Check sheet for the drawn part. Datum: minimum x, y, z corner. Units: mm. A direction names the side the tool comes from. Give positions to 0.01 mm unless a question says otherwise; leave off trailing zeros. Order: outer loops, then holes, each group sorted by start corner. A loop starts at its lowest first (then second) coordinate and runs counter-clockwise, first axis right, second up. Notation, with made-up numbers: M 35.25,38 L 81.25,38 A16 ccw 81.25,65 Z; hole C 50,-11.5 d1. An arc over 180 degrees is marked long. Answer as CSV lines item,"result". Start each with the question number.
Q1. Thickness scan on line 1 (Y direction, x = 70, z = 19); line 2 (X direction, y = 58, z = 49) (3 decimals); line 3 (Z direction, x = 15.5, y = 12.5). Record the ranges inside material, lowest first.
Q2. Section check C-C, the plane z = 19.05. Record the boundary of the cut face in (x, y) (1 decimal).
Q3. Section check B-B, the plane z = 34.5. Record the boundary of the cut face in (x, y) (3 decimals), then the cut area to 3 significant figures.
Q4. Go/stop test with flat-tipped pins: pin 1 (8 mm diameter, centred on y = 34.5, z = 32.5, fed in from -X); pin 2 (4 mm diameter, centred on x = 13, y = 20.5, fed in from -Z); pin 3 (22 mm diameter, centred on x = 29.5, y = 21, fed in from -Z) (3 decimals). Record where each tip stops, or that it passes through.
Q5. Mould release check, pull along Z, two halves, no side actions. Record for the marked faces 1, 2 and 3: +Z half, -Z half, draft (parallel to the pull), parting line (faces both ways), or undercut.
Q6. Section check A-A, the plane y = 31.75. Count the separate pieces of the cut face and the enclosed holes in it, then the cut area to 3 significant figures.
Q7. Set-up check for the marked faces 4 and 5: record each of +Z, -Z, +X, -X, +Y, -Y from which the full face is reachable in a straight line by a thin tool's end or side.
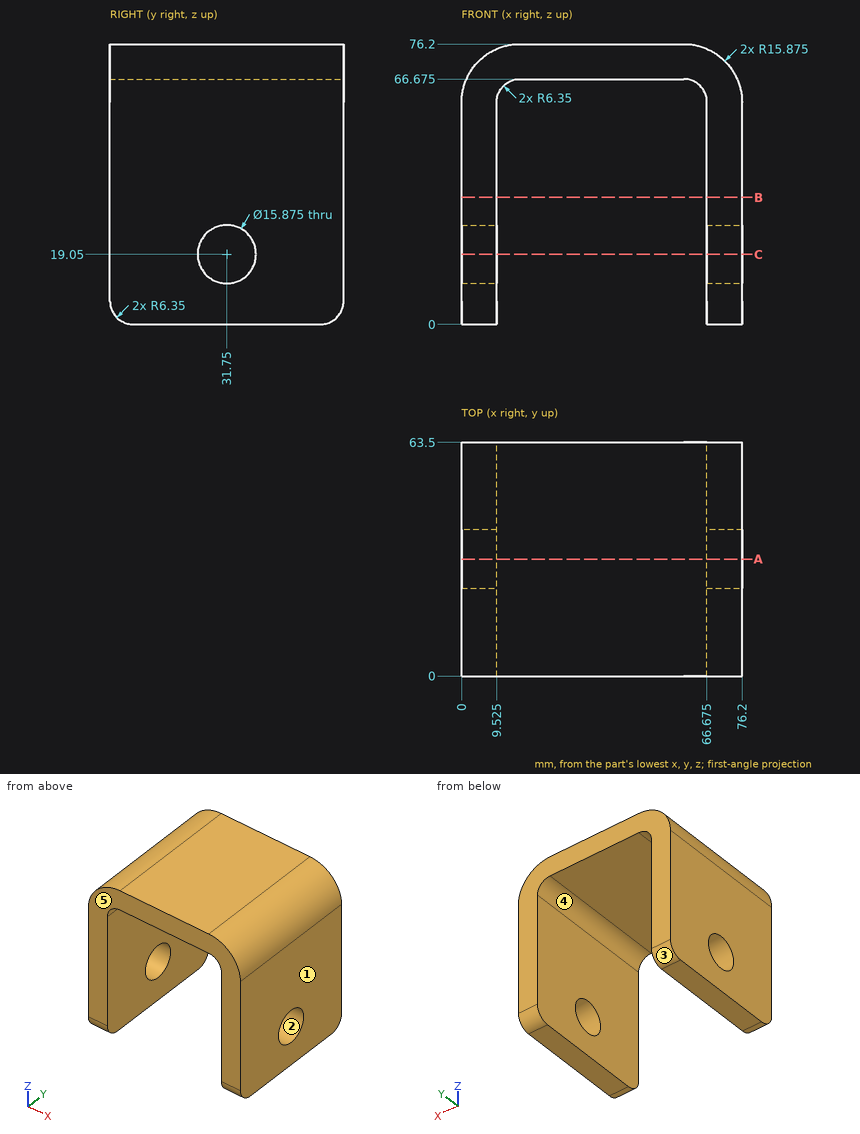
Answer block:
1,line 1,"y = 0 to 23.81, 39.69 to 63.5"
1,line 2,"x = 0 to 9.525, 66.675 to 76.2"
1,line 3,"z = 66.66 to 76.2"
2,outline,"M 0,0 L 9.5,0 L 9.5,23.8 L 0,23.8 Z; M 0,39.7 L 9.5,39.7 L 9.5,63.5 L 0,63.5 Z; M 66.7,0 L 76.2,0 L 76.2,23.8 L 66.7,23.8 Z; M 66.7,39.7 L 76.2,39.7 L 76.2,63.5 L 66.7,63.5 Z"
3,outline,"M 0,0 L 9.525,0 L 9.525,63.5 L 0,63.5 Z; M 66.675,0 L 76.2,0 L 76.2,63.5 L 66.675,63.5 Z"
3,area,"1,210 mm2"
4,pin 1,"stops at x = 0"
4,pin 2,"stops at z = 64.39"
4,pin 3,"stops at z = 66.675"
5,face 1,"draft"
5,face 2,"undercut"
5,face 3,"-Z half"
6,separate pieces,"3"
6,enclosed holes,"0"
6,area,"1,600 mm2"
7,face 4,"-Z, +Y, -Y"
7,face 5,"+Z, -Z, +X, -X, -Y"
